Design review of the part built by this model. Coordinates are the model's own, in mm. A direction names the side the tool comes from. Coordinates: 2 decimals unless noted, no trailing zeros. Order: outer loops, then holes, each group sorted by start corner. A loop starts at its lowest first (then second) coordinate and runs counter-clockwise, first axis right, second up. Notation, with made-up numbers: M -28,-2 L 17,-2 A17 cw 17,11 Z; hole C -9.5,65.5 d7. An arc over 180 degrees is marked long. Use CSV: the item, a comma, the result in double quotes.
```python
from build123d import *

# Parameters (mm, degrees)
SKETCH1_R           = 4.25
SKETCH1_W           = 2
SKETCH1_H           = 15
SKETCH1_W_2         = 20
SKETCH1_H_2         = 2
BOSS_EXTRUDE1_DEPTH = 4


with BuildPart() as part:
    # Sketch1 → Boss-Extrude1 (new body)
    with BuildSketch(Plane(origin=(0, 0, 0), x_dir=(1, 0, 0), z_dir=(0, 1, 0))):
        with BuildLine():
            Line((-161.5, -165), (161.5, -165))
            Line((161.5, -165), (161.5, -59.29))
            Line((161.5, -59.29), (216.5, -59.29))
            ThreePointArc((216.5, -59.29), (220.035533906, -57.825533906), (221.5, -54.29))
            Line((221.5, -54.29), (221.5, -47.29))
            Line((221.5, -47.29), (221.5, -40.29))
            ThreePointArc((221.5, -40.29), (220.035533906, -36.754466094), (216.5, -35.29))
            Line((216.5, -35.29), (161.5, -35.29))
            Line((161.5, -35.29), (161.5, 149.084720808))
            Line((161.5, 149.084720808), (205.651015663, 167.64799054))
            ThreePointArc((205.651015663, 167.64799054), (212.06200946, 183.361015663), (196.348984337, 189.77200946))
            Line((196.348984337, 189.77200946), (137.431056973, 165))
            Line((137.431056973, 165), (-137.431056973, 165))
            Line((-137.431056973, 165), (-196.348984337, 189.77200946))
            ThreePointArc((-196.348984337, 189.77200946), (-212.06200946, 183.361015663), (-205.651015663, 167.64799054))
            Line((-205.651015663, 167.64799054), (-161.5, 149.084720808))
            Line((-161.5, 149.084720808), (-161.5, -35.29))
            Line((-161.5, -35.29), (-216.5, -35.29))
            ThreePointArc((-216.5, -35.29), (-220.035533906, -36.754466094), (-221.5, -40.29))
            Line((-221.5, -40.29), (-221.5, -47.29))
            Line((-221.5, -47.29), (-221.5, -54.29))
            ThreePointArc((-221.5, -54.29), (-220.035533906, -57.825533906), (-216.5, -59.29))
            Line((-216.5, -59.29), (-161.5, -59.29))
            Line((-161.5, -59.29), (-161.5, -165))
        make_face()
        with Locations(Location((-201, -47.29, 0), (0, 0, 270))):
            Circle(SKETCH1_R, mode=Mode.SUBTRACT)
        with Locations(Location((201, -47.29, 0), (0, 0, 90))):
            Circle(SKETCH1_R, mode=Mode.SUBTRACT)
        with Locations(Location((-201, 178.71, 0), (0, 0, 270))):
            Circle(SKETCH1_R, mode=Mode.SUBTRACT)
        with Locations(Location((201, 178.71, 0), (0, 0, 270))):
            Circle(SKETCH1_R, mode=Mode.SUBTRACT)
        with Locations((155.5, 99)):
            Rectangle(SKETCH1_W, SKETCH1_H, mode=Mode.SUBTRACT)
        with Locations((155.5, 139)):
            Rectangle(SKETCH1_W, SKETCH1_H, mode=Mode.SUBTRACT)
        with Locations((155.5, 59)):
            Rectangle(SKETCH1_W, SKETCH1_H, mode=Mode.SUBTRACT)
        with Locations((155.5, 19)):
            Rectangle(SKETCH1_W, SKETCH1_H, mode=Mode.SUBTRACT)
        with Locations((90.5, 159)):
            Rectangle(SKETCH1_W_2, SKETCH1_H_2, mode=Mode.SUBTRACT)
        with Locations((135.5, 159)):
            Rectangle(SKETCH1_W_2, SKETCH1_H_2, mode=Mode.SUBTRACT)
        with Locations((45.5, 159)):
            Rectangle(SKETCH1_W_2, SKETCH1_H_2, mode=Mode.SUBTRACT)
        with Locations((-45.5, 159)):
            Rectangle(SKETCH1_W_2, SKETCH1_H_2, mode=Mode.SUBTRACT)
        with Locations((-135.5, 159)):
            Rectangle(SKETCH1_W_2, SKETCH1_H_2, mode=Mode.SUBTRACT)
        with Locations((-90.5, 159)):
            Rectangle(SKETCH1_W_2, SKETCH1_H_2, mode=Mode.SUBTRACT)
        with Locations((-155.5, 59)):
            Rectangle(SKETCH1_W, SKETCH1_H, mode=Mode.SUBTRACT)
        with Locations((-155.5, 19)):
            Rectangle(SKETCH1_W, SKETCH1_H, mode=Mode.SUBTRACT)
        with Locations((-155.5, 99)):
            Rectangle(SKETCH1_W, SKETCH1_H, mode=Mode.SUBTRACT)
        with Locations((-155.5, 139)):
            Rectangle(SKETCH1_W, SKETCH1_H, mode=Mode.SUBTRACT)
        with Locations((-155.5, -99)):
            Rectangle(SKETCH1_W, SKETCH1_H, mode=Mode.SUBTRACT)
        with Locations((-135.5, -159)):
            Rectangle(SKETCH1_W_2, SKETCH1_H_2, mode=Mode.SUBTRACT)
        with Locations((-155.5, -139)):
            Rectangle(SKETCH1_W, SKETCH1_H, mode=Mode.SUBTRACT)
        with Locations((-155.5, -59)):
            Rectangle(SKETCH1_W, SKETCH1_H, mode=Mode.SUBTRACT)
        with Locations((-155.5, -19)):
            Rectangle(SKETCH1_W, SKETCH1_H, mode=Mode.SUBTRACT)
        with Locations((-90.5, -159)):
            Rectangle(SKETCH1_W_2, SKETCH1_H_2, mode=Mode.SUBTRACT)
        with Locations((-45.5, -159)):
            Rectangle(SKETCH1_W_2, SKETCH1_H_2, mode=Mode.SUBTRACT)
        with Locations((155.5, -19)):
            Rectangle(SKETCH1_W, SKETCH1_H, mode=Mode.SUBTRACT)
        with Locations((155.5, -59)):
            Rectangle(SKETCH1_W, SKETCH1_H, mode=Mode.SUBTRACT)
        with Locations((155.5, -99)):
            Rectangle(SKETCH1_W, SKETCH1_H, mode=Mode.SUBTRACT)
        with Locations((155.5, -139)):
            Rectangle(SKETCH1_W, SKETCH1_H, mode=Mode.SUBTRACT)
        with Locations((135.5, -159)):
            Rectangle(SKETCH1_W_2, SKETCH1_H_2, mode=Mode.SUBTRACT)
        with Locations((90.5, -159)):
            Rectangle(SKETCH1_W_2, SKETCH1_H_2, mode=Mode.SUBTRACT)
        with Locations((45.5, -159)):
            Rectangle(SKETCH1_W_2, SKETCH1_H_2, mode=Mode.SUBTRACT)
        with Locations((104.5, -37)):
            Rectangle(SKETCH1_W_2, SKETCH1_H_2, mode=Mode.SUBTRACT)
        with Locations((44.5, -37)):
            Rectangle(SKETCH1_W_2, SKETCH1_H_2, mode=Mode.SUBTRACT)
        with Locations((-15.5, -37)):
            Rectangle(SKETCH1_W_2, SKETCH1_H_2, mode=Mode.SUBTRACT)
        with Locations((-75.5, -37)):
            Rectangle(SKETCH1_W_2, SKETCH1_H_2, mode=Mode.SUBTRACT)
        with Locations((-105.5, -80.5)):
            Rectangle(SKETCH1_W, SKETCH1_H, mode=Mode.SUBTRACT)
        with Locations((-105.5, -140.5)):
            Rectangle(SKETCH1_W, SKETCH1_H, mode=Mode.SUBTRACT)
        with Locations((-105.5, -115.5)):
            Rectangle(SKETCH1_W, SKETCH1_H, mode=Mode.SUBTRACT)
        with Locations((-105.5, -55.5)):
            Rectangle(SKETCH1_W, SKETCH1_H, mode=Mode.SUBTRACT)
    extrude(amount=BOSS_EXTRUDE1_DEPTH)


solid = part.part
```
(1) The part is to be moulded in two halves that separate along X. For faces 1 (the face through (-166.478, 1.972, -177.213)), 2 (the face through (183.27, 1.97, -158.24)), 3 (the face through (-183.885, 1.972, -158.496)), 4 (the face through (-3, 4, -15)), say which applies: pulls with the +X half, pulls with the -X half, needs draft (parallel to the pull), parting line crosses it, or undercut.
The answers:
face 1,"undercut"
face 2,"pulls with the +X half"
face 3,"pulls with the -X half"
face 4,"needs draft"
(2) Wall thickness on probe 1 along X at (y, z) = (3.1, 47.29); probe 2 along Z at (x, y) = (54, 3.05); probe 3 along X at (y, z) = (3.1, -65): over which ranges is each line inside the solid? List them lowest first.
The answers:
probe 1,"x = -221.5 to -205.25, -196.75 to 196.75, 205.25 to 221.5"
probe 2,"z = -165 to -160, -158 to 36, 38 to 158, 160 to 165"
probe 3,"x = -161.5 to -156.5, -154.5 to 154.5, 156.5 to 161.5"
(3) Add section C-C on z = 1. State the section outline as (x, y) points, and give its area (3 significant figures).
The answers:
outline,"M -161.5,0 L 161.5,0 L 161.5,4 L -161.5,4 Z"
area,"1,290 mm2"
(4) For faces 5 (the face through (-3, 0, -15)), 6 (the face through (167.3, 1.97, -177.56)), list the 3-axis set-ups (+Z, -Z, +X, -X, +Y, -Y) from which the entire face can be reached by the end or side of a thin tool; tool diameter is ignored.
The answers:
face 5,"+Z, -Z, +X, -X, -Y"
face 6,"-Z, +Y, -Y"
(5) Clearance check with flat-ended pins moving along their axes: P1, Ø1.5, axis at y = 3.5, z = -74.5, coming from the +X side; P2, Ø0.6, axis at y = 1, z = 159, coming from the -X side; P3, Ø1, axis at y = 3, z = 37, coming from the +X side; P4, Ø7, axis at x = 201, z = -178.71, coming from the -Y side. State where each tip first meets the part, or that it passes through.
The answers:
P1,"stops at x = 161.5"
P2,"stops at x = -161.5"
P3,"stops at x = 220.65"
P4,"passes through"
(6) Add section B-B on y = 0.75. Give the number of separate pieces and of enclosed holes in the cut face, and give its area (3 significant figures).
The answers:
separate pieces,"1"
enclosed holes,"40"
area,"111,000 mm2"
(7) Add section A-A on x = -91.5. State the section outline as (y, z) points, and give its area (3 significant figures).
The answers:
outline,"M 0,-165 L 4,-165 L 4,-160 L 0,-160 Z; M 0,-158 L 4,-158 L 4,158 L 0,158 Z; M 0,160 L 4,160 L 4,165 L 0,165 Z"
area,"1,300 mm2"
